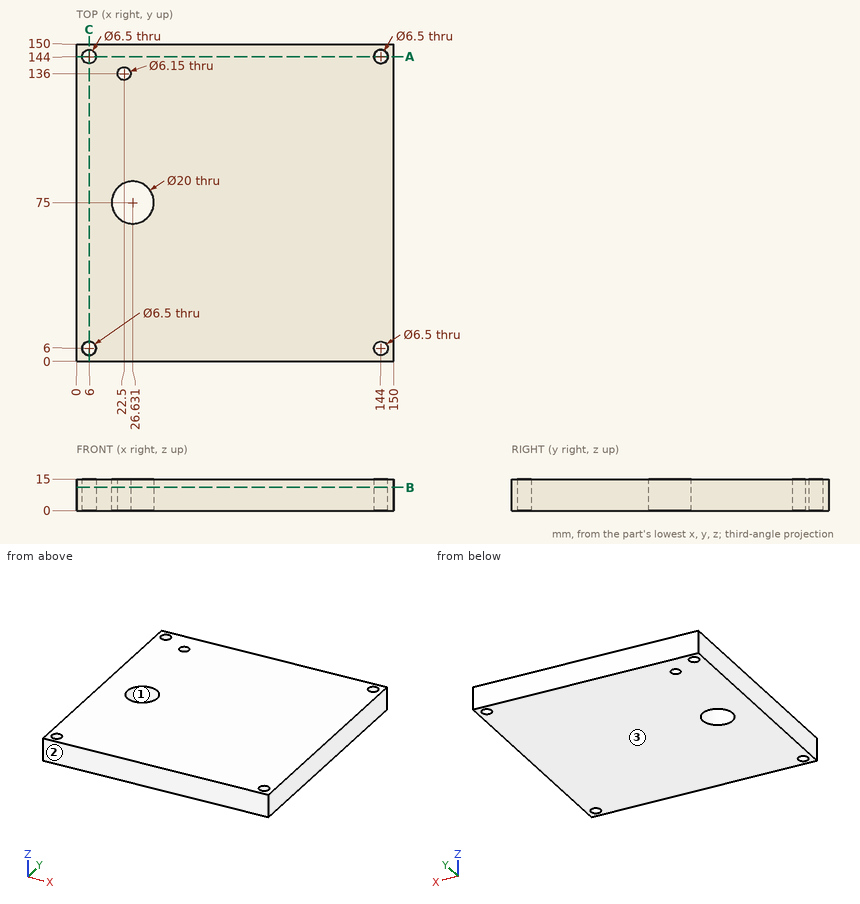
Can you work these out from the drawing? Everything is in mm from the part's minimum corner. Give positions to 0.01 mm unless a question says otherwise; leave off trailing zeros. Loops run counter-clockwise (first coordinate to the right, second up) from the corner with the lowest first, then second, coordinate; pieces in that order, holes last. Notation, with made-up numbers: (6, 73) - (11, 73) arc R20 cw to (11, 110) - close; hole circle Ø6 at (31, 39.5). An arc over 180 degrees is marked (long way). Use one line per item in the form item = value.
1. I want a section at A-A (y = 144). Please give me the cut outline in (x, z), and give its area (4 significant figures).
Response values:
outline = (0, 0) - (2.75, 0) - (2.75, 15) - (0, 15) - close; (9.25, 0) - (140.75, 0) - (140.75, 15) - (9.25, 15) - close; (147.25, 0) - (150, 0) - (150, 15) - (147.25, 15) - close
area = 2,055 mm²
2. Thinking about a two-plate mould opening in Y: for the marked faces 1, 2 and 3, which applies, released by +Y, released by -Y, zero draft, split by the parting line, or undercut?
Response values:
face_1 = undercut
face_2 = released by -Y
face_3 = zero draft
3. I need wall thicknesses on probe 1 along Y at (x, z) = (144, 9.5); probe 2 along X at (y, z) = (136, 10.25) (3 decimals). Which ranges of each line are inside material? Lowest first, please.
Response values:
probe_1 = 0 to 2.75, 9.25 to 140.75, 147.25 to 150
probe_2 = 0 to 19.425, 25.575 to 150
4. I want a section at B-B (z = 11). Please give me the cut outline in (x, y) (3 decimals).
Response values:
outline = (0, 0) - (150, 0) - (150, 150) - (0, 150) - close; hole circle Ø6.5 at (6, 6); hole circle Ø6.5 at (6, 144); hole circle Ø20 at (26.631, 75); hole circle Ø6.15 at (22.5, 136); hole circle Ø6.5 at (144, 6); hole circle Ø6.5 at (144, 144)
